Job drawing, mm, ordinate dimensions from the low corner. One solid piece. Round coordinates to 2 decimals unless told otherwise and drop trailing zeros. Order: outer loops, then holes, each group sorted by start corner. A loop starts at its lowest first (then second) coordinate and runs counter-clockwise, first axis right, second up. Notation, with made-up numbers: (70, 81) -> (74, 81) arc R13 ccw to (74, 85) -> close; hole circle Ø7 at (42.5, -22.75). An arc over 180 degrees is marked (long way). Return JSON: item names as keys, results as strings. Group by question number.
Q1. Probe line 1 along X through (y, z) = (1.3, 44.5); line 2 along X through (y, z) = (1.15, 12.5). List the from-to ranges inside material, lowest first.
Q2. Cut at C-C (z = 27). Write the cut outline in (x, y).
Q3. Cut at A-A (y = 0.7). Write the cut outline in (x, z), then the cut area to 3 significant figures.
Q4. Cut at B-B (z = 41). Write the cut outline in (x, y), then the cut area to 3 significant figures.
Q5. Flat gauge pins, fed straight in: pin 1 (2.5 mm diameter, centred on x = 65.5, z = 30, fed in from -Y); pin 2 (0.6 mm diameter, centred on y = 1, z = 42.5, fed in from -X); pin 3 (0.5 mm diameter, centred on x = 65, y = 1.5, fed in from +Z). Where does each tip first touch, or does it go through?
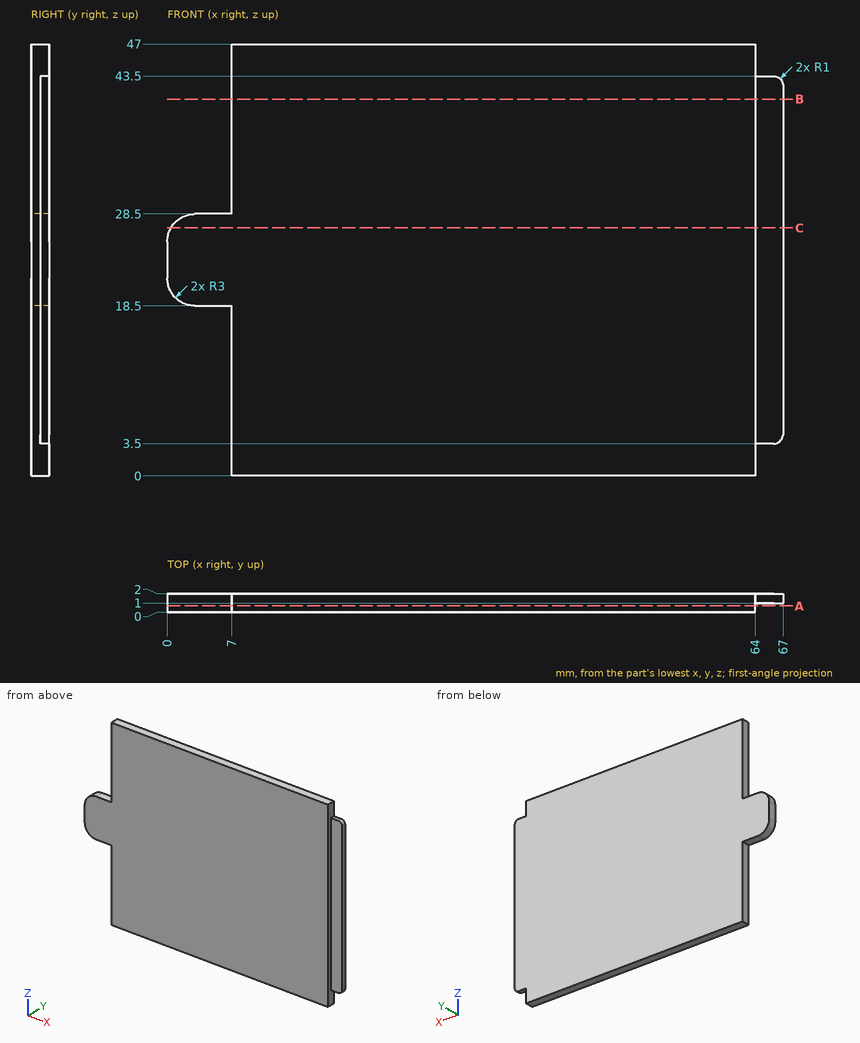
Solution:
{
 "1": {"line 1": "x = 7 to 64", "line 2": "x = 7 to 67"},
 "2": {"outline": "(0.4, 0) -> (64, 0) -> (64, 1) -> (67, 1) -> (67, 2) -> (0.4, 2) -> close"},
 "3": {"outline": "(0, 21.5) arc R3 ccw to (3, 18.5) -> (7, 18.5) -> (7, 0) -> (64, 0) -> (64, 47) -> (7, 47) -> (7, 28.5) -> (3, 28.5) arc R3 ccw to (0, 25.5) -> close", "area": "2,750 mm²"},
 "4": {"outline": "(7, 0) -> (64, 0) -> (64, 1) -> (67, 1) -> (67, 2) -> (7, 2) -> close", "area": "117 mm²"},
 "5": {"pin 1": "stops at y = 1", "pin 2": "stops at x = 7", "pin 3": "stops at z = 43.5"}
}
